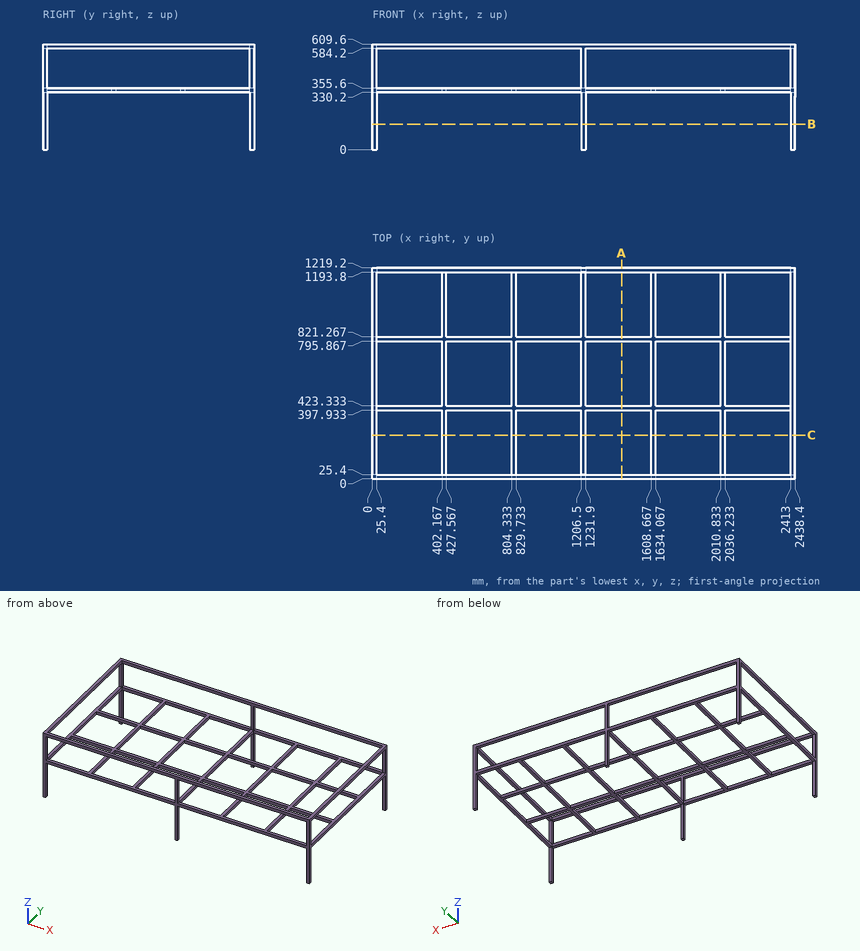
Source: three-view drawing plus pictorial views. Frame: mm from the lowest corner of the part. Coordinates: 2 decimals unless noted, no trailing zeros. Write each loop counter-clockwise with the first axis right and the second up, starting at its lowest first coordinate (ties: lowest second). Pieces come first, ordered by that corner, then holes. Notation, with made-up numbers: (4, 80) - (26, 80) arc R23 cw to (26, 91) - close; hole circle Ø2 at (-16, 18.5). An arc over 180 degrees is marked (long way). Return JSON: item names as keys, results as strings.
Item 1: Section query B-B (z = 147). Output: boundary loops of the cut face in (x, y).
Completed:
{"outline": "(0, 0) - (25.4, 0) - (25.4, 25.4) - (0, 25.4) - close; (0, 1193.8) - (25.4, 1193.8) - (25.4, 1219.2) - (0, 1219.2) - close; (1206.5, 0) - (1231.9, 0) - (1231.9, 25.4) - (1206.5, 25.4) - close; (1206.5, 1193.8) - (1231.9, 1193.8) - (1231.9, 1219.2) - (1206.5, 1219.2) - close; (2413, 0) - (2438.4, 0) - (2438.4, 25.4) - (2413, 25.4) - close; (2413, 1193.8) - (2438.4, 1193.8) - (2438.4, 1219.2) - (2413, 1219.2) - close"}
Item 2: Pin query (flat end, axial travel): pin 1 Ø20.5 at (x, y) = (17, 574.5) entering from -Z; pin 2 Ø6 at (x, y) = (971, 411) entering from +Z. Return the tip coordinate at first contact, or that it passes through.
Completed:
{"pin 1": "stops at z = 330.2", "pin 2": "stops at z = 355.6"}
Item 3: Line query: L1, parallel to Y at x = 1213.5, z = 570.5. Output: solid intervals per line, ascending.
Completed:
{"L1": "y = 0 to 25.4, 1193.8 to 1219.2"}
Item 4: Section query C-C (y = 252.5). Count the separate pieces of the cut face and the enclosed holes in it, and give its area (3 significant figures).
Completed:
{"separate pieces": "9", "enclosed holes": "0", "area": "5,810 mm2"}
Item 5: Section query A-A (x = 1437.5). Output: boundary loops of the cut face in (y, z), and give its area (3 significant figures).
Completed:
{"outline": "(0, 330.2) - (25.4, 330.2) - (25.4, 355.6) - (0, 355.6) - close; (0, 584.2) - (25.4, 584.2) - (25.4, 609.6) - (0, 609.6) - close; (397.93, 330.2) - (423.33, 330.2) - (423.33, 355.6) - (397.93, 355.6) - close; (795.87, 330.2) - (821.27, 330.2) - (821.27, 355.6) - (795.87, 355.6) - close; (1193.8, 330.2) - (1219.2, 330.2) - (1219.2, 355.6) - (1193.8, 355.6) - close; (1193.8, 584.2) - (1219.2, 584.2) - (1219.2, 609.6) - (1193.8, 609.6) - close", "area": "3,870 mm2"}
